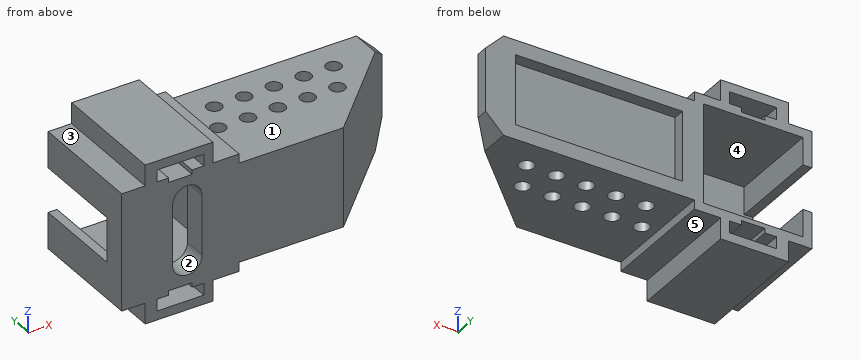
Autodesk Inventor part; units mm, degrees
ref_plane "YZ Plane" through (0, 0, 0) normal (1, 0, 0) x (0, 1, 0)
ref_plane "XZ Plane" through (0, 0, 0) normal (0, 1, 0) x (-1, 0, 0)
ref_plane "XY Plane" through (0, 0, 0) normal (0, 0, 1) x (1, 0, 0)
sketch "Sketch1" plane through (0, 0, 0) normal (0, 1, 0) x (-1, 0, 0)
  line L0 (0, 0) -> (50, 0)
  line L1 (50, 0) -> (50, -50)
  line L2 (50, -50) -> (0, -50)
  line L3 (0, -50) -> (0, 0)
  dimension "d0" = 50
extrude "Extrusion1" add sketch "Sketch1" along normal blind 10
sketch "Sketch2" plane through (0, 10, 0) normal (0, 1, 0) x (1, 0, 0)
  line L0 (0, 50) -> (-50, 50) construction
  line L1 (-50, 0) -> (0, 0) construction
  line L2 (0, 0) -> (0, 50) construction
  line L3 (-46.2, 46.2) -> (-3.8, 46.2)
  line L4 (-3.8, 46.2) -> (-3.8, 3.8)
  line L5 (-3.8, 3.8) -> (-46.2, 3.8)
  line L6 (0, 0) -> (-50, 0)
  line L7 (0, 0) -> (0, 50)
  line L8 (0, 50) -> (-50, 50)
  line L9 (-50, 50) -> (-50, 0) construction
  line L10 (-46.2, 34.5) -> (-46.2, 15.5)
  line L11 (-50, 50) -> (-50, 34.5)
  line L12 (-50, 34.5) -> (-46.2, 34.5)
  line L13 (-46.2, 34.5) -> (-46.2, 46.2)
  line L14 (-46.2, 0) -> (-50, 0)
  line L15 (-50, 0) -> (-50, 15.5)
  line L16 (-50, 15.5) -> (-46.2, 15.5)
  line L17 (-46.2, 15.5) -> (-46.2, 3.8)
  point P0 (0, 25)
  point P1 (-3.8, 25)
  point P2 (-25, 46.2)
  point P3 (-25, 50)
  point P4 (-46.2, 50)
  point P5 (-46.2, 25)
  dimension "d6" = 42.4
  dimension "d7" = 42.4
  dimension "d10" = 19
  dimension "d11" = 3.8
extrude "Extrusion2" add sketch "Sketch2" along normal blind 39.5 contours L13 L12 L11 L8 L7 L6 L15 L16 L17 L5 L4 L3
sketch "Sketch3" plane through (0, 49.5, 0) normal (0, 1, 0) x (1, 0, 0)
  line L0 (0, 0) -> (0, 50) construction
  line L1 (0, 50) -> (-50, 50) construction
  line L2 (-46.2, 46.2) -> (-3.8, 46.2) construction
  line L3 (-20, 50) -> (-20, 48.095)
  line L4 (-20, 48.095) -> (-30, 48.095)
  line L5 (-30, 48.095) -> (-30, 50)
  line L6 (-30, 50) -> (-20, 50)
  line L7 (0, 25) -> (-50, 25)
  line L8 (-50, 34.5) -> (-50, 15.5) construction
  line L9 (0, 0) -> (-50, 0) construction
  line L10 (-46.2, 3.8) -> (-3.8, 3.8) construction
  line L11 (-20, 0) -> (-20, 1.905)
  line L12 (-20, 1.905) -> (-30, 1.905)
  line L13 (-30, 1.905) -> (-30, 0)
  line L14 (-30, 0) -> (-20, 0)
  point P0 (-25, 48.095)
  point P1 (-25, 50)
  point P2 (-25, 1.905)
  point P3 (-25, 0)
  dimension "d12" = 1.905
  dimension "d13" = 10
extrude "Extrusion3" cut sketch "Sketch3" against normal through all
sketch "Sketch4" plane through (0, 49.5, 0) normal (0, 1, 0) x (1, 0, 0)
  line L0 (-3.8, 46.2) -> (-3.8, 3.8) construction
  line L1 (0, 0) -> (0, 50) construction
  line L2 (0, 3.85) -> (88.9, 3.85)
  line L3 (88.9, 3.85) -> (88.9, 46.15)
  line L4 (88.9, 46.15) -> (0, 46.15)
  line L5 (0, 3.85) -> (0, 46.15)
  point P0 (-3.8, 25)
  point P1 (88.9, 25)
  dimension "d16" = 88.9
  dimension "d17" = 42.3
extrude "Extrusion4" add sketch "Sketch4" against normal blind 49.5
chamfer "Chamfer1" distance 7.62 angle 45 2 edges at (88.9, 24.75, -3.85) (88.9, 24.75, -46.15)
chamfer "Chamfer2" distance 44.45 angle 45 1 edges at (88.9, 0, -25)
sketch "Sketch5" plane through (0, 0, -3.85) normal (0, 0, 1) x (1, 0, 0)
  line L0 (0, 49.5) -> (81.28, 49.5) construction
  line L1 (0, 0) -> (0, 49.5) construction
  circle A0 centre (12.7, 36.8) radius 3.175
  circle A1 centre (25.4, 36.8) radius 3.175
  circle A2 centre (38.1, 36.8) radius 3.175
  circle A3 centre (50.8, 36.8) radius 3.175
  circle A4 centre (63.5, 36.8) radius 3.175
  circle A5 centre (6.35, 24.1) radius 3.175
  circle A6 centre (19.05, 24.1) radius 3.175
  circle A7 centre (31.75, 24.1) radius 3.175
  circle A8 centre (44.45, 24.1) radius 3.175
  circle A9 centre (57.15, 24.1) radius 3.175
  dimension "d26" = 6.35
  dimension "d27" = 12.7
  dimension "d28" = 12.7
  dimension "d29" = 12.7
  dimension "d30" = 12.7
  dimension "d31" = 12.7
  dimension "d32" = 12.7
  dimension "d33" = 6.35
  dimension "d34" = 12.7
  dimension "d35" = 12.7
  dimension "d36" = 12.7
  dimension "d37" = 12.7
  dimension "d38" = 12.7
  dimension "d39" = 6.35
extrude "Extrusion5" cut sketch "Sketch5" against normal through all
sketch "Sketch6" plane through (0, 49.5, 0) normal (0, 1, 0) x (1, 0, 0)
  line L0 (88.9, 11.47) -> (88.9, 38.53) construction
  line L1 (76.2, 10.0775) -> (5.08, 10.0775)
  line L2 (5.08, 10.0775) -> (5.08, 39.9225)
  line L3 (5.08, 39.9225) -> (76.2, 39.9225)
  line L4 (76.2, 39.9225) -> (76.2, 10.0775)
  point P0 (76.2, 25)
  point P1 (88.9, 25)
  dimension "d42" = 71.12
  dimension "d43" = 29.845
  dimension "d44" = 12.7
extrude "Extrusion6" cut sketch "Sketch6" against normal blind 5
sketch "Sketch7" plane through (0, 49.5, 0) normal (0, 1, 0) x (1, 0, 0)
  line L0 (-20, 50) -> (-20, 48.095) construction
  line L1 (-30, 48.095) -> (-30, 50) construction
  line L2 (-30, 50) -> (-50, 50) construction
  line L3 (-3.8, 46.2) -> (-3.8, 3.8) construction
  line L4 (-50, 0) -> (-30, 0) construction
  line L5 (-30, 0) -> (-30, 1.905) construction
  line L6 (-30, 1.905) -> (-20, 1.905) construction
  line L7 (-20, 0) -> (0, 0) construction
  line L8 (-34.98, -5.08) -> (-15.02, -5.08)
  line L9 (-34.98, 0) -> (-34.98, -5.08)
  line L10 (-15.02, 0) -> (-15.02, -5.08)
  line L11 (-11.21, 0) -> (-11.21, -8.89)
  line L12 (-11.21, -8.89) -> (-40, -8.89)
  line L13 (-40, -8.89) -> (-40, 0)
  line L14 (-50, 34.5) -> (-50, 15.5) construction
  line L15 (-50, 25) -> (-3.8, 25)
  line L16 (-15.02, 50) -> (-15.02, 55.08)
  line L17 (-34.98, 55.08) -> (-15.02, 55.08)
  line L18 (-34.98, 50) -> (-34.98, 55.08)
  line L19 (-11.21, 50) -> (-11.21, 58.89)
  line L20 (-11.21, 58.89) -> (-40, 58.89)
  line L21 (-40, 58.89) -> (-40, 50)
  line L22 (-50, 0) -> (-30, 0) construction
  line L23 (-40, 0) -> (-34.98, 0)
  line L24 (-15.02, 0) -> (-11.21, 0)
  line L25 (-11.21, 50) -> (-15.02, 50)
  line L26 (-34.98, 50) -> (-40, 50)
  point P0 (-25, 1.905)
  point P1 (-25, -5.08)
  point P2 (-25, 55.08)
  dimension "d49" = 5.08
  dimension "d50" = 19.96
  dimension "d52" = 3.81
  dimension "d53" = 3.81
extrude "Extrusion7" add sketch "Sketch7" against normal blind 49.5
sketch "Sketch8" plane through (0, 0, 0) normal (0, -1, 0) x (1, 0, 0)
  line L0 (-50, -50) -> (-50, 0) construction
  line L1 (-22.06, -37.7) -> (-22.06, -12.3) construction
  line L2 (-28.41, -37.7) -> (-28.41, -12.3)
  line L3 (-15.71, -12.3) -> (-15.71, -37.7)
  arc A0 (-28.41, -37.7) -> (-15.71, -37.7) centre (-22.06, -37.7) ccw
  arc A1 (-15.71, -12.3) -> (-28.41, -12.3) centre (-22.06, -12.3) ccw
  point P0 (-22.06, -25)
  point P1 (-50, -25)
  dimension "d56" = 12.7
  dimension "d57" = 21.59
  dimension "d58" = 25.4
extrude "Extrusion8" cut sketch "Sketch8" against normal blind 25.4
properties part number "StepperMotorHolder"
Here's how the part is built. I have some questions about the finished solid (model axes, mm). Face numbers are marked on the shaded views. A direction names the side the tool comes from. Give positions to 0.01 mm unless a question says otherwise; leave off trailing zeros. Loops run counter-clockwise (first coordinate to the right, second up) from the corner with the lowest first, then second, coordinate; pieces in that order, holes last. Notation, with made-up numbers: (13, 55) -> (68, 55) arc R24 cw to (68, 77) -> close; hole circle Ø4 at (-10, 72). An arc over 180 degrees is marked (long way). Answer as a JSON object with one key per item and string values. Group by question number.
Item 1: Will these pins go through, and if not, where does the flat tip stop? pin 1 (10 mm diameter, centred on x = 6.35, y = 24.1, fed in from -Z); pin 2 (5.5 mm diameter, centred on x = -3.5, y = 19, fed in from -Z); pin 3 (5 mm diameter, centred on x = -47, y = 31.5, fed in from +Z).
Item 2: I need wall thicknesses on L1, parallel to Z at x = -21.5, y = 15.5 (3 decimals); L2, parallel to Z at x = -31, y = 42; L3, parallel to X at y = 26, z = -19. Which ranges of each line are inside material? Lowest first, please.
Item 3: On a 3-axis mill with a long thin cutter (end or side, diameter ignored), from which of +Z, -Z, +X, -X, +Y, -Y can I reach the whole of each face in a straight line? I mean the marked faces 1, 2, 3, 4 and 5. Say none if no direction works.
Item 4: Imagine slicing it at A-A on z = -17. Give the number of separate pieces and of enclosed holes in the cut face, then the cut area to 3 significant figures.
Item 5: Imagine slicing it at C-C on x = -13. Write out the boundary of the cut face in (y, z), then the cut area to 3 significant figures.
Answer list:
{
 "1": {"pin 1": "stops at z = -46.15", "pin 2": "stops at z = -50", "pin 3": "stops at z = 0"},
 "2": {"L1": "z = -58.89 to -55.08, -48.095 to -46.2, -3.8 to -1.905, 5.08 to 8.89", "L2": "z = -58.89 to -55.08, -50 to -46.2, -3.8 to 0, 5.08 to 8.89", "L3": "x = -3.8 to 3.81, 8.89 to 16.51, 21.59 to 29.21, 34.29 to 41.91, 46.99 to 54.61, 59.69 to 70.45"},
 "3": {"face 1": "+Z, +X, +Y, -Y", "face 2": "+Y, -Y", "face 3": "+Z, -X, +Y, -Y", "face 4": "+Y", "face 5": "-Z, +X, +Y, -Y"},
 "4": {"separate pieces": "2", "enclosed holes": "10", "area": "3,260 mm2"},
 "5": {"outline": "(0, -58.89) -> (49.5, -58.89) -> (49.5, -46.2) -> (10, -46.2) -> (10, -3.8) -> (49.5, -3.8) -> (49.5, 8.89) -> (0, 8.89) -> close", "area": "1,680 mm2"}
}
